```python
from build123d import *

# Parameters (mm, degrees)
SKETCH_W      = 40
SKETCH_H      = 40
SKETCH_R      = 5
EXTRUDE_DEPTH = 5


with BuildPart() as part:
    # Sketch → Extrude (new body)
    with BuildSketch(Plane.XY):
        Rectangle(SKETCH_W, SKETCH_H)
        Circle(SKETCH_R, mode=Mode.SUBTRACT)
    extrude(amount=EXTRUDE_DEPTH)


solid = part.part
```
Verification items for the finished model (mm, model axes). Round coordinates to 2 decimals unless told otherwise and drop trailing zeros. Write each loop counter-clockwise with the first axis right and the second up, starting at its lowest first coordinate (ties: lowest second). Pieces come first, ordered by that corner, then holes.
1. Section check A-A on x = 0. Enter the section's corners in (y, z).
2. Draft check along Y on faces 1 (the flat face through (0, -20, 2)), 2 (the flat face through (-5, -4, 5)), 3 (the cylindrical face through (-1.08, -4.88, 2.46)). Enter one of: +Y half, -Y half, draft (parallel to the pull), parting line (faces both ways), or undercut.
3. Section check C-C on z = 2.85. Enter the section's corners in (x, y), plus the area to 3 significant figures.
4. Scan lines: L1, parallel to Y at x = 0, z = 3.45; L2, parallel to X at y = -3.5, z = 1.75; L3, parallel to Y at x = -4, z = 1.7. Record each from-to range of solid material in increasing order.
5. Section check B-B on y = -3. Enter the section's corners in (x, z), plus the area to 3 significant figures.
Answer:
1. outline: (-20, 0) - (-5, 0) - (-5, 5) - (-20, 5) - close; (5, 0) - (20, 0) - (20, 5) - (5, 5) - close
2. face 1: -Y half
2. face 2: draft
2. face 3: undercut
3. outline: (-20, -20) - (20, -20) - (20, 20) - (-20, 20) - close; hole circle Ø10 at (0, 0)
3. area: 1,520 mm2
4. L1: y = -20 to -5, 5 to 20
4. L2: x = -20 to -3.57, 3.57 to 20
4. L3: y = -20 to -3, 3 to 20
5. outline: (-20, 0) - (-4, 0) - (-4, 5) - (-20, 5) - close; (4, 0) - (20, 0) - (20, 5) - (4, 5) - close
5. area: 160 mm2
